```python
from build123d import *

# Parameters (mm, degrees)
F0_W     = 80
F0_H     = 70
F1_DEPTH = 50
F2_R     = 2.5
F3_DEPTH = 15
F4_R     = 8.5
F5_DEPTH = 92.7
F4_R_2   = 14
F6_DEPTH = 35
F4_R_3   = 2.5
F7_DEPTH = 20


with BuildPart() as f1:
    # F0 (on Top) → F1 (new body)
    with BuildSketch(Plane.XY):
        with Locations((1.460786, 3.671486)):
            Rectangle(F0_W, F0_H)
    extrude(amount=F1_DEPTH)

    # F2 (on face) → F3 (cut)
    with BuildSketch(Plane.XY.offset(50)):
        with Locations((-28.539214, 33.671486)):
            Circle(F2_R)
        with Locations((-28.481222, -26.328486)):
            Circle(F2_R)
        with Locations((31.460602, 33.522883)):
            Circle(F2_R)
        with Locations((31.518594, -26.477089)):
            Circle(F2_R)
    extrude(amount=-F3_DEPTH, mode=Mode.SUBTRACT)

    # F4 (on face) → F5 (cut)
    with BuildSketch(Plane.YZ.offset(41.460786)):
        with Locations((3.671486, 29.85)):
            Circle(F4_R)
    extrude(amount=-F5_DEPTH, mode=Mode.SUBTRACT)

    # F4 (on face) → F6 (cut)
    with BuildSketch(Plane.YZ.offset(41.460786)):
        with Locations((3.671486, 29.85)):
            Circle(F4_R_2)
        with Locations((3.671486, 29.85)):
            Circle(F4_R, mode=Mode.SUBTRACT)
    extrude(amount=-F6_DEPTH, mode=Mode.SUBTRACT)

    # F4 (on face) → F7 (cut)
    with BuildSketch(Plane.YZ.offset(41.460786)):
        with Locations((-6.309632, 46.017167)):
            Circle(F4_R_3)
        with Locations((-15.328514, 29.85)):
            Circle(F4_R_3)
        with Locations((-6.309632, 13.682833)):
            Circle(F4_R_3)
        with Locations((13.652604, 13.682833)):
            Circle(F4_R_3)
        with Locations((22.671486, 29.85)):
            Circle(F4_R_3)
        with Locations((13.652604, 46.017167)):
            Circle(F4_R_3)
    extrude(amount=-F7_DEPTH, mode=Mode.SUBTRACT)


solid = f1.part
```
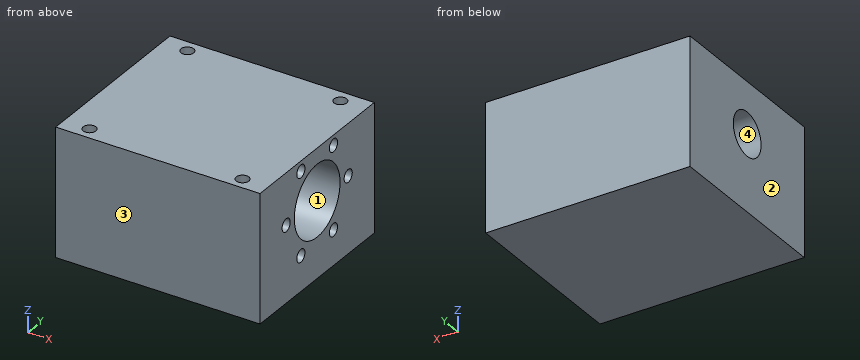
Part model, mm, in its own coordinate system. Face numbers are marked on the shaded views. Give positions to 0.01 mm unless a question says otherwise; leave off trailing zeros. Loops run counter-clockwise (first coordinate to the right, second up) from the corner with the lowest first, then second, coordinate; pieces in that order, holes last. Notation, with made-up numbers: M 58,38.25 L 94,38.25 A29 cw 94,63.25 Z; hole C -2.75,-39 d10. An arc over 180 degrees is marked long. Return JSON: item names as keys, results as strings.
1) Flat gauge pins, fed straight in: pin 1 Ø2.5 at (y, z) = (-7, 47) entering from +X; pin 2 Ø2.5 at (x, y) = (-29, -26.5) entering from +Z. Where does each tip first touch, or does it go through?
Calculated:
{"pin 1": "stops at x = 21.46", "pin 2": "stops at z = 35"}
2) Saw through at D-D, the plane x = -24.5. List the corners of the cut face in (y, z), then the cut area to 3 significant figures.
Calculated:
{"outline": "M -31.33,0 L 38.67,0 L 38.67,50 L -31.33,50 Z; hole C 3.67,29.85 d17", "area": "3,270 mm2"}
3) Pull direction Y, two halves, no side cores. Call the marked faces 1, 2, 3 and 4: released by +Y, released by -Y, zero draft, split by the parting line, or undercut.
Calculated:
{"face 1": "undercut", "face 2": "zero draft", "face 3": "released by -Y", "face 4": "undercut"}
4) Saw through at C-C, the plane x = 35. List the corners of the cut face in (y, z), then the cut area to 3 significant figures.
Calculated:
{"outline": "M -31.33,0 L 38.67,0 L 38.67,50 L -31.33,50 Z; hole C -15.33,29.85 d5; hole C 3.67,29.85 d28; hole C -6.31,13.68 d5; hole C -6.31,46.02 d5; hole C 13.65,13.68 d5; hole C 13.65,46.02 d5; hole C 22.67,29.85 d5", "area": "2,770 mm2"}
5) Drill centre lines: line 1 (Z direction, x = -4, y = 3); line 2 (Y direction, x = -30.5, z = 22.5); line 3 (Z direction, x = -14.5, y = -1). Where is each one in solid material? Low to high.
Calculated:
{"line 1": "z = 0 to 21.38, 38.32 to 50", "line 2": "y = -31.33 to -0.6, 7.94 to 38.67", "line 3": "z = 0 to 22.75, 36.95 to 50"}
6) Saw through at B-B, the plane z = 36. List the corners of the cut face in (x, y).
Calculated:
{"outline": "M -38.54,-31.33 L 41.46,-31.33 L 41.46,-8.91 L 6.46,-8.91 L 6.46,-2.2 L -38.54,-2.2 Z; M -38.54,9.54 L 6.46,9.54 L 6.46,16.25 L 41.46,16.25 L 41.46,38.67 L -38.54,38.67 Z; hole C -28.54,33.67 d5; hole C -28.48,-26.33 d5; hole C 31.46,33.52 d5; hole C 31.52,-26.48 d5"}
7) Saw through at A-A, the plane z = 29.85. List the corners of the cut face in (x, y).
Calculated:
{"outline": "M -38.54,-31.33 L 41.46,-31.33 L 41.46,-17.83 L 21.46,-17.83 L 21.46,-12.83 L 41.46,-12.83 L 41.46,-10.33 L 6.46,-10.33 L 6.46,-4.83 L -38.54,-4.83 Z; M -38.54,12.17 L 6.46,12.17 L 6.46,17.67 L 41.46,17.67 L 41.46,20.17 L 21.46,20.17 L 21.46,25.17 L 41.46,25.17 L 41.46,38.67 L -38.54,38.67 Z"}
